Build history of the part. All positions in model axes, mm. Face numbers are marked on the shaded views. A direction names the side the tool comes from. Round coordinates to 2 decimals unless told otherwise and drop trailing zeros. Loops run counter-clockwise (first coordinate to the right, second up) from the corner with the lowest first, then second, coordinate; pieces in that order, holes last.
from build123d import *

# Parameters (mm, degrees)
SKETCH1_W            = 36
SKETCH1_H            = 24.25
BOSS_EXTRUDE1_DEPTH  = 1.6
SKETCH2_R            = 1.875
CUT_EXTRUDE1_DEPTH   = 39.020726256
FILLET1_R            = 3
SKETCH3_W            = 12
SKETCH3_H            = 12
BOSS_EXTRUDE2_DEPTH  = 3.8
SKETCH4_R            = 3.4
BOSS_EXTRUDE3_DEPTH  = 3
SKETCH5_R            = 6.5
BOSS_EXTRUDE4_DEPTH  = 1.25
SKETCH6_R            = 5.75
BOSS_EXTRUDE5_DEPTH  = 4
FILLET2_R            = 0.5
SKETCH7_W            = 2.5
SKETCH7_H            = 7.5
BOSS_EXTRUDE6_DEPTH  = 2.55
SKETCH8_W            = 0.65
SKETCH8_H            = 0.65
BOSS_EXTRUDE7_DEPTH  = 5.75
BOSS_EXTRUDE8_DEPTH  = 7.85
CUT_EXTRUDE2_DEPTH   = 6.2
SKETCH11_W           = 3.15
SKETCH11_H           = 6.75
CUT_EXTRUDE3_DEPTH   = 1
SKETCH12_W           = 1.25
SKETCH12_H           = 6.75
CUT_EXTRUDE4_DEPTH   = 0.6
SKETCH13_W           = 1.5
SKETCH13_H           = 3.45
BOSS_EXTRUDE9_DEPTH  = 0.75
SKETCH14_W           = 1.15
SKETCH14_H           = 0.75
CUT_EXTRUDE5_DEPTH   = 4.5
SKETCH15_W           = 1
SKETCH15_H           = 1
BOSS_EXTRUDE10_DEPTH = 1.6
SKETCH16_W           = 0.75
SKETCH16_H           = 0.75
BOSS_EXTRUDE11_DEPTH = 2


with BuildPart() as part:
    # Sketch1 → Boss-Extrude1 (new body)
    with BuildSketch(Plane(origin=(0, 0, 0), x_dir=(1, 0, 0), z_dir=(0, 1, 0))):
        with Locations((18, 0)):
            Rectangle(SKETCH1_W, SKETCH1_H)
    extrude(amount=BOSS_EXTRUDE1_DEPTH)

    # Sketch2 → Cut-Extrude1 (cut, through all)
    with BuildSketch(Plane(origin=(0, 1.6, 0), x_dir=(1, 0, 0), z_dir=(0, 1, 0))):
        with Locations(Location((31.975, 8, 0), (0, 0, 270))):
            Circle(SKETCH2_R)
        with Locations(Location((31.975, -8, 0), (0, 0, 270))):
            Circle(SKETCH2_R)
    extrude(amount=-CUT_EXTRUDE1_DEPTH, mode=Mode.SUBTRACT)

    # Fillet1
    fillet1_edges = [part.edges().sort_by_distance(p)[0] for p in [
        (36, 0.8, -12.125),
        (36, 0.8, 12.125),
    ]]
    fillet(fillet1_edges, radius=FILLET1_R)

    # Sketch3 → Boss-Extrude2 (add)
    with BuildSketch(Plane(origin=(0, 1.6, 0), x_dir=(1, 0, 0), z_dir=(0, 1, 0))):
        with Locations((22, 0)):
            Rectangle(SKETCH3_W, SKETCH3_H)
    extrude(amount=BOSS_EXTRUDE2_DEPTH)

    # Sketch4 → Boss-Extrude3 (add)
    with BuildSketch(Plane(origin=(0, 5.4, 0), x_dir=(1, 0, 0), z_dir=(0, 1, 0))):
        with Locations(Location((22, 0, 0), (0, 0, 270))):
            Circle(SKETCH4_R)
    extrude(amount=BOSS_EXTRUDE3_DEPTH)

    # Sketch5 → Boss-Extrude4 (add)
    with BuildSketch(Plane(origin=(0, 8.4, 0), x_dir=(1, 0, 0), z_dir=(0, 1, 0))):
        with Locations(Location((22, 0, 0), (0, 0, 270))):
            Circle(SKETCH5_R)
    extrude(amount=BOSS_EXTRUDE4_DEPTH)

    # Sketch6 → Boss-Extrude5 (add)
    with BuildSketch(Plane(origin=(0, 9.65, 0), x_dir=(1, 0, 0), z_dir=(0, 1, 0))):
        with Locations(Location((22, 0, 0), (0, 0, 270))):
            Circle(SKETCH6_R)
    extrude(amount=BOSS_EXTRUDE5_DEPTH)

    # Fillet2
    fillet2_edges = [part.edges().sort_by_distance(p)[0] for p in [
        (22, 13.65, -5.75),
    ]]
    fillet(fillet2_edges, radius=FILLET2_R)

    # Sketch7 → Boss-Extrude6 (add)
    with BuildSketch(Plane(origin=(0, 1.6, 0), x_dir=(1, 0, 0), z_dir=(0, 1, 0))):
        with Locations((5.05, -6.525)):
            Rectangle(SKETCH7_W, SKETCH7_H)
    extrude(amount=BOSS_EXTRUDE6_DEPTH)

    # Sketch8 → Boss-Extrude7 (add)
    with BuildSketch(Plane.ZY.offset(-3.8)):
        with Locations((4.075, 2.875)):
            Rectangle(SKETCH8_W, SKETCH8_H)
        with Locations((6.525, 2.875)):
            Rectangle(SKETCH8_W, SKETCH8_H)
        with Locations((8.975, 2.875)):
            Rectangle(SKETCH8_W, SKETCH8_H)
    extrude(amount=BOSS_EXTRUDE7_DEPTH)

    # Sketch9 → Boss-Extrude8 (add)
    with BuildSketch(Plane.ZY.offset(-0.25)):
        Polygon((-9.025, 1.6), (1.075, 1.6), (1.075, 6.8), (-0.6, 6.8), (-0.6, 5.95), (-7.35, 5.95), (-7.35, 6.8), (-9.025, 6.8), align=None)
    extrude(amount=-BOSS_EXTRUDE8_DEPTH)

    # Sketch10 → Cut-Extrude2 (cut)
    with BuildSketch(Plane.ZY.offset(-0.25)):
        Polygon((-8.425, 6.2), (-8.425, 2.2), (0.475, 2.2), (0.475, 6.2), (0, 6.2), (0, 5.35), (-7.95, 5.35), (-7.95, 6.2), align=None)
    extrude(amount=-CUT_EXTRUDE2_DEPTH, mode=Mode.SUBTRACT)

    # Sketch11 → Cut-Extrude3 (cut)
    with BuildSketch(Plane(origin=(0, 5.95, 0), x_dir=(1, 0, 0), z_dir=(0, 1, 0))):
        with Locations((1.825, 3.975)):
            Rectangle(SKETCH11_W, SKETCH11_H)
    extrude(amount=-CUT_EXTRUDE3_DEPTH, mode=Mode.SUBTRACT)

    # Sketch12 → Cut-Extrude4 (cut)
    with BuildSketch(Plane(origin=(0, 2.2, 0), x_dir=(1, 0, 0), z_dir=(0, 1, 0))):
        with Locations((0.875, 3.975)):
            Rectangle(SKETCH12_W, SKETCH12_H)
    extrude(amount=-CUT_EXTRUDE4_DEPTH, mode=Mode.SUBTRACT)

    # Sketch13 → Boss-Extrude9 (add)
    with BuildSketch(Plane(origin=(0, 5.95, 0), x_dir=(1, 0, 0), z_dir=(0, 1, 0))):
        with Locations((4.15, 3.975)):
            Rectangle(SKETCH13_W, SKETCH13_H)
    extrude(amount=BOSS_EXTRUDE9_DEPTH)

    # Sketch14 → Cut-Extrude5 (cut)
    with BuildSketch(Plane(origin=(0, 5.95, 0), x_dir=(1, 0, 0), z_dir=(0, 1, 0))):
        with Locations((7.525, 6.975)):
            Rectangle(SKETCH14_W, SKETCH14_H)
        with Locations((7.525, 4.975)):
            Rectangle(SKETCH14_W, SKETCH14_H)
        with Locations((7.525, 2.975)):
            Rectangle(SKETCH14_W, SKETCH14_H)
        with Locations((7.525, 0.975)):
            Rectangle(SKETCH14_W, SKETCH14_H)
    extrude(amount=-CUT_EXTRUDE5_DEPTH, mode=Mode.SUBTRACT)

    # Sketch15 → Boss-Extrude10 (add)
    with BuildSketch(Plane.XZ):
        with Locations((24.5, -6.1)):
            Rectangle(SKETCH15_W, SKETCH15_H)
        with Locations((19.5, 6.1)):
            Rectangle(SKETCH15_W, SKETCH15_H)
        with Locations((24.5, 6.1)):
            Rectangle(SKETCH15_W, SKETCH15_H)
        with Locations((19.5, -6.1)):
            Rectangle(SKETCH15_W, SKETCH15_H)
    extrude(amount=BOSS_EXTRUDE10_DEPTH)

    # Sketch16 → Boss-Extrude11 (add)
    with BuildSketch(Plane.XZ):
        with Locations((7.625, 8.95)):
            Rectangle(SKETCH16_W, SKETCH16_H)
        with Locations((7.625, 6.45)):
            Rectangle(SKETCH16_W, SKETCH16_H)
        with Locations((7.625, 3.95)):
            Rectangle(SKETCH16_W, SKETCH16_H)
        with Locations((7.625, -0.65)):
            Rectangle(SKETCH16_W, SKETCH16_H)
        with Locations((7.625, -2.8)):
            Rectangle(SKETCH16_W, SKETCH16_H)
        with Locations((7.625, -4.95)):
            Rectangle(SKETCH16_W, SKETCH16_H)
        with Locations((7.625, -7.1)):
            Rectangle(SKETCH16_W, SKETCH16_H)
    extrude(amount=BOSS_EXTRUDE11_DEPTH)


solid = part.part
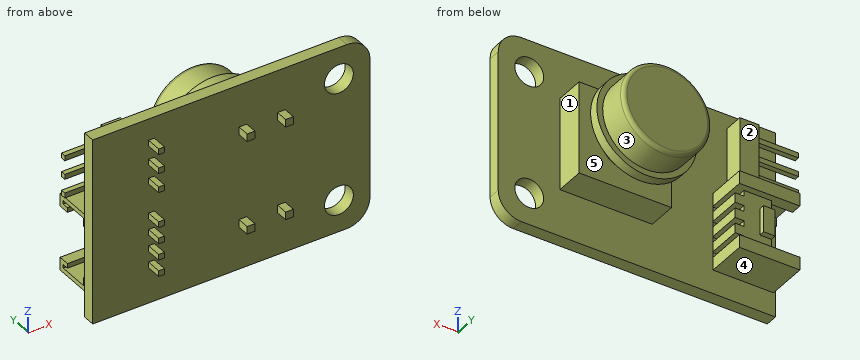
(1) Which spindle directions (+Z, -Z, +X, -X, +Y, -Y) get a long thin tool onto all of the face, cutting with end or side? Do the marked faces 1, 2, 3, 4 and 5. Say none if no direction does.
Responses:
face 1: +Z, -Z, +X
face 2: +Z, -X, +Y
face 3: +Y
face 4: -Z, +X, -X, +Y
face 5: none
(2) Slice it at B-B on z = 8. List the corners of the cut face in (x, y), plus the area to 3 significant figures.
Responses:
outline: (0, 0) - (30.1, 0) - (30.1, 1.6) - (6.3, 1.6) - (6.3, 4.15) - (3.8, 4.15) - (3.8, 1.6) - (0, 1.6) - close; (33.85, 0) - (36, 0) - (36, 1.6) - (33.85, 1.6) - close
area: 58.0 mm2
(3) Slice it at C-C on x = 22. List the corners of the cut face in (y, z) (3 decimals).
Responses:
outline: (0, -12.125) - (1.6, -12.125) - (1.6, -6) - (5.4, -6) - (5.4, -3.4) - (8.4, -3.4) - (8.4, -6.5) - (9.65, -6.5) - (9.65, -5.75) - (13.15, -5.75) arc R0.5 ccw to (13.65, -5.25) - (13.65, 5.25) arc R0.5 ccw to (13.15, 5.75) - (9.65, 5.75) - (9.65, 6.5) - (8.4, 6.5) - (8.4, 3.4) - (5.4, 3.4) - (5.4, 6) - (1.6, 6) - (1.6, 12.125) - (0, 12.125) - close
(4) Slice it at D-D on y = 7.75. List the corners of the cut face in (x, z), plus the area to 3 significant figures.
Responses:
outline: circle Ø6.8 at (22, 0)
area: 36.3 mm2
(5) Slice it at A-A on x = 3. Count the separate pieces of the cut face and the enclosed holes in it, plus the area to 3 significant figures.
Responses:
separate pieces: 4
enclosed holes: 0
area: 54.0 mm2
(6) Probe line 1 (X direction, y = 1, z = 8); line 2 (X direction, y = 4.5, z = 0.25); line 3 (Y direction, x = 25.5, z = 3.5). List the from-to ranges inside material, lowest first.
Responses:
line 1: x = 0 to 30.1, 33.85 to 36
line 2: x = 6.45 to 8.1, 16 to 28
line 3: y = 0 to 5.4, 8.4 to 13.65
(7) Pin check, flat tips, straight feed: P1, Ø0.6, axis at y = -0.5, z = 4, coming from the -X side; P2, Ø8, axis at y = 10, z = -4.5, coming from the +X side; P3, Ø0.6, axis at x = 7.5, y = -1, coming from the -Z side (3 decimals). Stop position of each tip, or through.
Responses:
P1: stops at x = 7.25
P2: stops at x = 28.48
P3: stops at z = -7.475
